Design review of the part shown in the three views and the two pictorial views. Dimensions are in mm from the part's minimum x, y and z. A direction names the side the tool comes from. Round coordinates to 2 decimals unless told otherwise and drop trailing zeros. Order: outer loops, then holes, each group sorted by start corner. A loop starts at its lowest first (then second) coordinate and runs counter-clockwise, first axis right, second up.
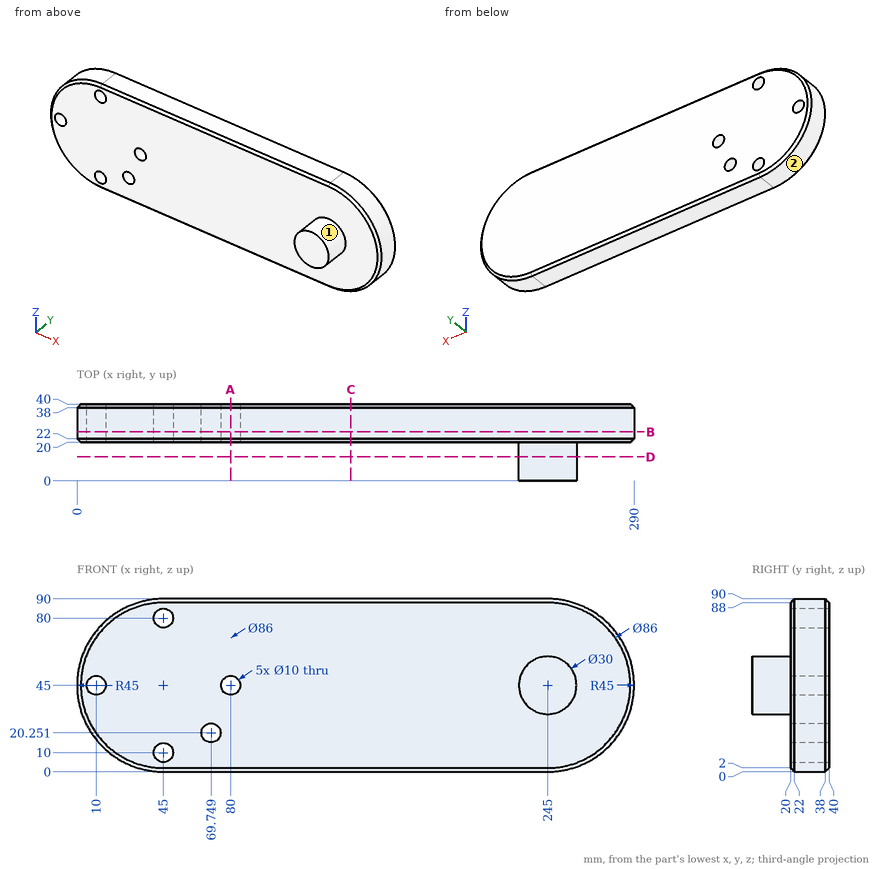
(1) Add section A-A on x = 80. Give the boundary of the cut face in (y, z), plus the area to 3 significant figures.
(2) Tool access review of the marked faces 1 and 2: name each direction out of +Z, -Z, +X, -X, +Y, -Y from which nothing blocks a thin tool from reaching the whole face with its end or side.
(3) Clearance check with a flat-ended pin moving along its axis: P1, Ø4, axis at y = 28.5, z = 25, coming from the +X side. State where the tip first meets the part, or that it passes through.
(4) Wall thickness on L1, parallel to X at y = 25, z = 45; L2, parallel to Z at x = 45, y = 32.75; L3, parallel to Z at x = 79.5, y = 23.5 (1 decimal): over which ranges is each line inside the solid? List them lowest first.
(5) Add section D-D on y = 12.5. Give the boundary of the cut face in (x, z), plus the area to 3 significant figures.
(6) Add section B-B on y = 25.5. Give the boundary of the cut face in (x, z).
(7) Add section C-C on x = 142.5. Give the boundary of the cut face in (y, z).
Here are the results:
1. outline: (20, 2) - (22, 0) - (38, 0) - (40, 2) - (40, 40) - (20, 40) - close; (20, 50) - (40, 50) - (40, 88) - (38, 90) - (22, 90) - (20, 88) - close
1. area: 1,590 mm2
2. face 1: -Y
2. face 2: -X, +Y, -Y
3. P1: stops at x = 286.24
4. L1: x = 0 to 5, 15 to 75, 85 to 290
4. L2: z = 0 to 5, 15 to 75, 85 to 90
4. L3: z = 0 to 40, 50 to 90
5. outline: circle Ø30 at (245, 45)
5. area: 707 mm2
6. outline: (45, 0) - (245, 0) arc R45 ccw to (245, 90) - (45, 90) arc R45 ccw to start; hole circle Ø10 at (10, 45); hole circle Ø10 at (45, 10); hole circle Ø10 at (45, 80); hole circle Ø10 at (69.75, 20.25); hole circle Ø10 at (80, 45)
7. outline: (20, 2) - (22, 0) - (38, 0) - (40, 2) - (40, 88) - (38, 90) - (22, 90) - (20, 88) - close
